Check sheet for the modelled part. Datum: model origin and axes. Units: mm. Face numbers are marked on the shaded views. A direction names the side the tool comes from. Round coordinates to 2 decimals unless told otherwise and drop trailing zeros. Loops run counter-clockwise (first coordinate to the right, second up) from the corner with the lowest first, then second, coordinate; pieces in that order, holes last. Notation, with made-up numbers: (-30, 1.25) - (19, 1.25) arc R9 cw to (19, 15.25) - close; hole circle Ø2 at (71.25, 63.25). An arc over 180 degrees is marked (long way). Return JSON: item names as keys, results as strings.
Autodesk Inventor part; units mm, degrees
ref_plane "YZ Plane" through (0, 0, 0) normal (1, 0, 0) x (0, 1, 0)
ref_plane "XZ Plane" through (0, 0, 0) normal (0, 1, 0) x (-1, 0, 0)
ref_plane "XY Plane" through (0, 0, 0) normal (0, 0, 1) x (1, 0, 0)
sketch "スケッチ1" plane through (0, 0, 0) normal (0, 0, 1) x (1, 0, 0)
  circle A0 centre (0, 0) radius 7.5
  dimension "DIA" = 15
extrude "押し出し1" add sketch "スケッチ1" along normal blind 2
sketch "スケッチ2" plane through (0, 0, 2) normal (0, 0, 1) x (1, 0, 0)
  line L0 (0, 0) -> (0, 15)
  line L1 (0, 0) -> (-12.9904, 7.5)
  line L2 (0, 0) -> (15, 0) construction
  line L3 (-12.9904, 7.5) -> (0, 15)
  circle A0 centre (0, 0) radius 3
  point P0 (-2.5981, 1.5)
  point P1 (0, 3)
  dimension "d3" = 15
  dimension "d4" = 15
  dimension "d5" = 150
  dimension "HUB_DIA" = 6
extrude "押し出し2" cut sketch "スケッチ2" against normal blind 2 contours A0 L1 L3 L0
pattern_circular "円形状パターン1" count 3 over 360 about axis through (0, 0, -10) along (0, 0, 1) of "押し出し2"
sketch "スケッチ3" plane through (0, 0, 0) normal (0, 0, -1) x (-1, 0, 0)
  circle A0 centre (0, 0) radius 3
  arc A1 (0, -3) -> (2.5981, -1.5) centre (0, 0) ccw
extrude "押し出し3" add sketch "スケッチ3" along normal blind 2
sketch "スケッチ4" plane through (0, 0, -2) normal (0, 0, -1) x (-1, 0, 0)
  point P0 (0, 0)
  point P1 (0, 0)
hole "穴1" at (0, 0, -2) direction (0, 0, 1) diameter 2 end through all
equation "\"d3\" = DIA"
equation "\"d4\" = DIA"
equation "\"d6\" = THIN"
equation "\"d12\" = THIN"
properties part number "SlitDisc-FA130"
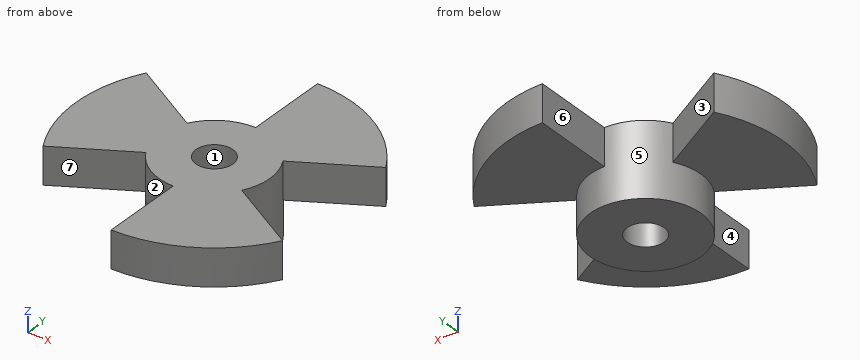
Q1. Sectioned sample at D-D (x = 2). Enter the section's corners in (y, z).
Answer key:
{"outline": "(-7.23, 0) - (-2.24, 0) - (-2.24, -2) - (2.24, -2) - (2.24, 0) - (7.23, 0) - (7.23, 2) - (-7.23, 2) - close"}
Q2. Scan lines: probe 1 along X at (y, z) = (0, -0.95); probe 2 along X at (y, z) = (0, 0.2); probe 3 along Z at (x, y) = (-4.5, 0.25). Record each from-to range of solid material in increasing order. Write a range as [from, to].
Answer key:
{"probe 1": "x = [-3, -1], [1, 3]", "probe 2": "x = [-7.5, -1], [1, 3]", "probe 3": "z = [0, 2]"}
Q3. Tool access check on the marked faces 5, 6 and 7. Record the directions out of +Z, -Z, +X, -X, +Y, -Y that give a thin tool (end or side, any length) a straight path to the whole face; none if there is none.
Answer key:
{"face 5": "-Z", "face 6": "+Z, -Z, +Y", "face 7": "+Z, -Z, -Y"}
Q4. Sectioned sample at B-B (z = 0.35). Enter the section's corners in (x, y), plus the area to 3 significant figures.
Answer key:
{"outline": "(-6.5, -3.75) - (-2.6, -1.5) arc R3 ccw to (0, -3) - (0, -7.5) arc R7.5 ccw to (6.5, -3.75) - (2.6, -1.5) arc R3 ccw to (2.6, 1.5) - (6.5, 3.75) arc R7.5 ccw to (0, 7.5) - (0, 3) arc R3 ccw to (-2.6, 1.5) - (-6.5, 3.75) arc R7.5 ccw to start; hole circle Ø2 at (0, 0)", "area": "99.4 mm²"}
Q5. Draft check along Y on the marked faces 1, 2, 3 and 4. Enter one of: released by +Y, released by -Y, zero draft, split by the parting line, or undercut.
Answer key:
{"face 1": "undercut", "face 2": "released by -Y", "face 3": "released by +Y", "face 4": "zero draft"}
Q6. Sectioned sample at A-A (y = 0). Enter the section's corners in (x, z), plus the area to 3 significant figures.
Answer key:
{"outline": "(-7.5, 0) - (-3, 0) - (-3, -2) - (-1, -2) - (-1, 2) - (-7.5, 2) - close; (1, -2) - (3, -2) - (3, 2) - (1, 2) - close", "area": "25.0 mm²"}
Q7. Depth check by flat-ended pin: P1, Ø2, axis at y = 4.5, z = 0.5, coming from the -X side; P2, Ø1, axis at y = -5, z = 1.5, coming from the -X side; P3, Ø5, axis at x = 2.5, y = 5, coming from the -Z side. Enter the tip coordinate at first touch or a pass-through.
Answer key:
{"P1": "stops at x = -6.63", "P2": "stops at x = 0", "P3": "stops at z = 0"}
Q8. Sectioned sample at C-C (x = 3.5). Enter the section's corners in (y, z).
Answer key:
{"outline": "(-6.63, 0) - (-2.02, 0) - (-2.02, 2) - (-6.63, 2) - close; (2.02, 0) - (6.63, 0) - (6.63, 2) - (2.02, 2) - close"}
